```python
from build123d import *

# Parameters (mm, degrees)
BOSS_EXTRUDE1_DEPTH = 10
FILLET1_R           = 1
CHAMFER1_SIZE       = 0.5


with BuildPart() as part:
    # Sketch1 → Boss-Extrude1 (new body)
    with BuildSketch(Plane(origin=(0, 0, 0), x_dir=(1, 0, 0), z_dir=(0, 1, 0))):
        Polygon((2.19, 0), (4.19, 0), (5.39, 2.3), (5.39, 4.3), (4.19, 4.3), (4.19, 6.29), (6.062127702, 6.29), (9.46014997, 9.086335224), (9.46014997, 15.100590628), (5.402376873, 18.882324593), (-3.212376873, 18.882324593), (-7.27014997, 15.100590628), (-7.27014997, 9.086335224), (-3.872127702, 6.29), (-2, 6.29), (-2, 4.3), (-3.2, 4.3), (-3.2, 2.3), (-2, 0), (0, 0), (0, 8.29), (-3.155, 8.29), (-5.27014997, 10.030620837), (-5.27014997, 14.230620837), (-2.424891086, 16.882324593), (4.614891086, 16.882324593), (7.46014997, 14.230620837), (7.46014997, 10.030620837), (5.345, 8.29), (2.19, 8.29), align=None)
    extrude(amount=BOSS_EXTRUDE1_DEPTH)

    # Fillet1
    fillet1_edges = [part.edges().sort_by_distance(p)[0] for p in [
        (5.345, 5, -8.29),
        (7.46014997, 5, -10.030620837),
        (7.46014997, 5, -14.230620837),
        (4.614891086, 5, -16.882324593),
        (-2.424891086, 5, -16.882324593),
        (-5.27014997, 5, -14.230620837),
        (-5.27014997, 5, -10.030620837),
        (-3.155, 5, -8.29),
        (0, 5, -8.29),
        (-3.872127702, 5, -6.29),
        (-7.27014997, 5, -9.086335224),
        (-7.27014997, 5, -15.100590628),
        (-3.212376873, 5, -18.882324593),
        (5.402376873, 5, -18.882324593),
        (9.46014997, 5, -15.100590628),
        (9.46014997, 5, -9.086335224),
        (6.062127702, 5, -6.29),
        (2.19, 5, -8.29),
    ]]
    fillet(fillet1_edges, radius=FILLET1_R)

    # Chamfer1
    chamfer1_edges = [part.edges().sort_by_distance(p)[0] for p in [
        (9.364426343, 0, -9.131530446),
        (9.377152184, 0, -15.064487844),
        (5.375000217, 0, -18.812795323),
        (-3.185000217, 0, -18.812795323),
        (-7.187152184, 0, -15.064487844),
        (-0.292893219, 0, -7.997106781),
        (-3.851086274, 0, -6.348682512),
        (-7.174426343, 0, -9.131530446),
        (-7.27014997, 10, -12.112041882),
        (4.088218075, 10, -8.29),
        (2.19, 10, -3.645),
        (4.946781925, 10, -6.29),
        (7.71728843, 10, -7.652081788),
        (9.46014997, 10, -12.112041882),
        (7.416178096, 10, -17.005516722),
        (1.095, 10, -18.882324593),
        (-5.226178096, 10, -17.005516722),
        (-2.756781925, 10, -6.29),
        (0, 10, -3.645),
        (-1.898218075, 10, -8.29),
        (-4.168724579, 10, -9.124224594),
        (-5.27014997, 10, -12.149199793),
        (-3.832435203, 10, -15.570531827),
        (1.095, 10, -16.882324593),
        (6.022435203, 10, -15.570531827),
        (7.46014997, 10, -12.149199793),
        (6.358724579, 10, -9.124224594),
        (2.482893219, 10, -7.997106781),
        (6.041086274, 10, -6.348682512),
        (9.364426343, 10, -9.131530446),
        (9.377152184, 10, -15.064487844),
        (5.375000217, 10, -18.812795323),
        (-3.185000217, 10, -18.812795323),
        (-7.187152184, 10, -15.064487844),
        (-0.292893219, 10, -7.997106781),
        (-3.851086274, 10, -6.348682512),
        (-7.174426343, 10, -9.131530446),
        (3.19, 10, 0),
        (-3.133958573, 0, -8.348682512),
        (-3.133958573, 10, -8.348682512),
        (-5.174426343, 0, -10.075816059),
        (-5.174426343, 10, -10.075816059),
        (-5.187152184, 0, -14.194518054),
        (-5.187152184, 10, -14.194518054),
        (-2.39751443, 0, -16.812795323),
        (-2.39751443, 10, -16.812795323),
        (4.58751443, 0, -16.812795323),
        (4.58751443, 10, -16.812795323),
        (5.323958573, 0, -8.348682512),
        (5.323958573, 10, -8.348682512),
        (7.364426343, 0, -10.075816059),
        (7.364426343, 10, -10.075816059),
        (7.377152184, 0, -14.194518054),
        (7.377152184, 10, -14.194518054),
        (4.79, 10, -1.15),
        (5.39, 10, -3.3),
        (4.79, 10, -4.3),
        (4.19, 10, -5.295),
        (-1, 0, 0),
        (-2.6, 0, -1.15),
        (-3.2, 0, -3.3),
        (-2.6, 0, -4.3),
        (-2, 0, -5.295),
        (4.19, 0, -5.295),
        (4.79, 0, -4.3),
        (5.39, 0, -3.3),
        (4.79, 0, -1.15),
        (3.19, 0, 0),
        (-2, 10, -5.295),
        (-2.6, 10, -4.3),
        (-3.2, 10, -3.3),
        (-2.6, 10, -1.15),
        (-1, 10, 0),
        (-5.52728843, 0, -7.652081788),
        (-5.52728843, 10, -7.652081788),
        (4.088218075, 0, -8.29),
        (6.358724579, 0, -9.124224594),
        (7.46014997, 0, -12.149199793),
        (6.022435203, 0, -15.570531827),
        (1.095, 0, -16.882324593),
        (-3.832435203, 0, -15.570531827),
        (-5.27014997, 0, -12.149199793),
        (-4.168724579, 0, -9.124224594),
        (-1.898218075, 0, -8.29),
        (0, 0, -3.645),
        (-2.756781925, 0, -6.29),
        (-7.27014997, 0, -12.112041882),
        (-5.226178096, 0, -17.005516722),
        (1.095, 0, -18.882324593),
        (7.416178096, 0, -17.005516722),
        (9.46014997, 0, -12.112041882),
        (7.71728843, 0, -7.652081788),
        (4.946781925, 0, -6.29),
        (2.19, 0, -3.645),
        (2.482893219, 0, -7.997106781),
        (6.041086274, 0, -6.348682512),
    ]]
    chamfer(chamfer1_edges, length=CHAMFER1_SIZE)


solid = part.part
```
Verification items for the finished model (mm, model axes). A direction names the side the tool comes from. Coordinates: 2 decimals unless noted, no trailing zeros. Loops run counter-clockwise (first coordinate to the right, second up) from the corner with the lowest first, then second, coordinate; pieces in that order, holes last. Notation, with made-up numbers: (-11.75, -31.5) - (38.25, -31.5) arc R18 ccw to (38.25, -4.5) - close; hole circle Ø6 at (13.25, 75). An arc over 180 degrees is marked (long way). Put each result on its own line as item: value.
Item 1: Gauge pin test, flat ends, axial feed: pin 1 Ø2 at (y, z) = (6, -3.5) entering from +X; pin 2 Ø1.7 at (x, y) = (5.5, 3) entering from +Z; pin 3 Ø1.5 at (y, z) = (2.5, -2) entering from -X. Record the tip position at first contact, or that the pin passes through.
Conclusion:
pin 1: stops at x = 5.39
pin 2: stops at z = -0.88
pin 3: stops at x = -3.2
Item 2: Set-up check for faces 1 (the face through (-3.8, 4.9, -15.6)), 2 (the face through (-3.2, 5, -3)), 3 (the face through (6.175, 0.254, -15.765)): record each of +Z, -Z, +X, -X, +Y, -Y from which the full face is reachable in a straight line by a thin tool's end or side.
Conclusion:
face 1: +Y, -Y
face 2: +Z, -X, +Y, -Y
face 3: -Y
Item 3: Section check A-A (z = -12.5). Enter the section's corners in (x, y).
Conclusion:
outline: (-7.27, 0.5) - (-6.77, 0) - (-5.77, 0) - (-5.27, 0.5) - (-5.27, 9.5) - (-5.77, 10) - (-6.77, 10) - (-7.27, 9.5) - close; (7.46, 0.5) - (7.96, 0) - (8.96, 0) - (9.46, 0.5) - (9.46, 9.5) - (8.96, 10) - (7.96, 10) - (7.46, 9.5) - close
Item 4: Section check C-C (z = -16). Enter the section's corners in (x, y).
Conclusion:
outline: (-6.31, 0.5) - (-5.57, 0) - (-4.1, 0) - (-3.37, 0.5) - (-3.37, 9.5) - (-4.1, 10) - (-5.57, 10) - (-6.31, 9.5) - close; (5.56, 0.5) - (6.29, 0) - (7.76, 0) - (8.5, 0.5) - (8.5, 9.5) - (7.76, 10) - (6.29, 10) - (5.56, 9.5) - close
Item 5: Scan lines: line 1 along X through (y, z) = (5.75, -10.5); line 2 along X through (y, z) = (8.75, -2.75); line 3 along Z through (x, y) = (-3, 5.5). Record each from-to range of solid material in increasing order.
Conclusion:
line 1: x = -7.27 to -5.27, 7.46 to 9.46
line 2: x = -3.2 to 0, 2.19 to 5.39
line 3: z = -18.87 to -16.35, -8.31 to -6.29, -4.3 to -1.92
Item 6: Section check B-B (x = 0.25). Enter the section's corners in (y, z).
Conclusion:
outline: (0, -18.38) - (0.5, -18.88) - (9.5, -18.88) - (10, -18.38) - (10, -17.38) - (9.5, -16.88) - (0.5, -16.88) - (0, -17.38) - close
Item 7: Draft check along Z on faces 4 (the face through (2.491, 5.063, -8.005)), 5 (the face through (7.27, 0.25, -16.8)), 6 (the face through (9.46, 5, -12)), 7 (the face through (-2, 5, -5)). Enter one of: pulls with the +Z half, pulls with the -Z half, needs draft (parallel to the pull), parting line crosses it, or undercut.
Conclusion:
face 4: undercut
face 5: pulls with the -Z half
face 6: needs draft
face 7: undercut
